Input: part model. Units: mm. Frame: model coordinates. Face numbers are marked on the shaded views. A direction names the side the tool comes from. Round coordinates to 2 decimals unless told otherwise and drop trailing zeros. Loops run counter-clockwise (first coordinate to the right, second up) from the corner with the lowest first, then second, coordinate; pieces in that order, holes last. Notation, with made-up numbers: (12, 27.5) -> (62, 27.5) arc R9 cw to (62, 40.5) -> close; hole circle Ø6 at (29, 66.5). An arc over 180 degrees is marked (long way). Answer as a JSON object with one key per item and string values. Group by question number.
Item 1: Draft query along Z for the marked faces 1, 2 and 3. Return one class per face: released by +Z, released by -Z, zero draft, split by the parting line, or undercut.
Item 2: Section query A-A on z = 0. Return loops of the section in (x, y).
Item 3: Pin query (flat end, axial travel): pin 1 (3 mm diameter, centred on y = 0, z = 0, fed in from -X); pin 2 (2 mm diameter, centred on x = 1, z = 6.5, fed in from -Y); pin 3 (1.5 mm diameter, centred on x = 1, z = -0.5, fed in from +Y); pin 4 (3 mm diameter, centred on x = 3.5, z = -7.5, fed in from +Y). Return the tip coordinate at first contact, or that it passes through.
Item 4: Material intervals for line 1 (Y direction, x = 1.6, z = 0); line 2 (Z direction, x = 2.75, y = -12); line 3 (Y direction, x = 3.3, z = 14), sorted ascending. Write a range as [from, to].
Item 5: Set-up query: the marked faces 4, 5 and 6. Return all of +Z, -Z, +X, -X, +Y, -Y with unobstructed straight access to the full face (end or side cutting, diameter ignored); none if empty.
from build123d import *

# Parameters (mm, degrees)
BASPROSKE_W        = 5
BASPROSKE_H        = 16
TOOTHCUT_DEPTH     = 24.173260453
TEETHCUTS_COUNT    = 30
TEETHCUTS_ANGLE    = 348
BORSKE_R           = 2.5
BORE_DEPTH         = 50.0000508
ESQUISSE1_R        = 3.356867485
BOSS_EXTRU_1_DEPTH = 5


with BuildPart() as part:
    # BasProSke → Base-Revolve (revolve)
    with BuildSketch(Plane(origin=(0, 0, 0), x_dir=(1, 0, 0), z_dir=(0, 1, 0)), mode=Mode.PRIVATE) as base_revolve_sk:
        with Locations((2.5, 8)):
            Rectangle(BASPROSKE_W, BASPROSKE_H)
    revolve(base_revolve_sk.sketch.rotate(Axis((-10, 0, 0), (1, 0, 0)), 180), axis=Axis((-10, 0, 0), (1, 0, 0)))

    # TooCutSke → ToothCut (cut, through all)
    with BuildSketch(Plane(origin=(0, 0, 0), x_dir=(0, 0, -1), z_dir=(1, 0, 0))):
        with BuildLine():
            ThreePointArc((0.466400716, 13.741086979), (0, 13.749), (-0.466400716, 13.741086979))
            ThreePointArc((-0.466400716, 13.741086979), (-0.819142092, 14.899954875), (-1.3974676, 15.964351834))
            ThreePointArc((-1.3974676, 15.964351834), (0, 16.0254), (1.3974676, 15.964351834))
            ThreePointArc((1.3974676, 15.964351834), (0.819142092, 14.899954875), (0.466400716, 13.741086979))
        make_face()
    toothcut = extrude(amount=TOOTHCUT_DEPTH, mode=Mode.SUBTRACT)

    # TeethCuts: ToothCut ×30 about axis
    teethcuts_axis = Axis((-10, 0, 0), (1, 0, 0))
    for i in range(1, TEETHCUTS_COUNT):
        add(toothcut.rotate(teethcuts_axis, i * TEETHCUTS_ANGLE / (TEETHCUTS_COUNT - 1)), mode=Mode.SUBTRACT)

    # BorSke → Bore (cut, symmetric)
    with BuildSketch(Plane(origin=(0, 0, 0), x_dir=(0, 0, -1), z_dir=(1, 0, 0))):
        with Locations(Location((0, 0, 0), (0, 0, 180))):
            Circle(BORSKE_R)
    extrude(amount=BORE_DEPTH, both=True, mode=Mode.SUBTRACT)

    # Esquisse1 → Boss.-Extru.1 (add)
    with BuildSketch(Plane(origin=(5, 0, 0), x_dir=(0, 0, -1), z_dir=(1, 0, 0))):
        Circle(ESQUISSE1_R)
        with BuildLine():
            Line((1.989182734, -1.514315704), (2.010613168, 1.485743817))
            ThreePointArc((2.010613168, 1.485743817), (-2.499936218, 0.017857885), (1.989182734, -1.514315704))
        make_face(mode=Mode.SUBTRACT)
    extrude(amount=-BOSS_EXTRU_1_DEPTH)


solid = part.part
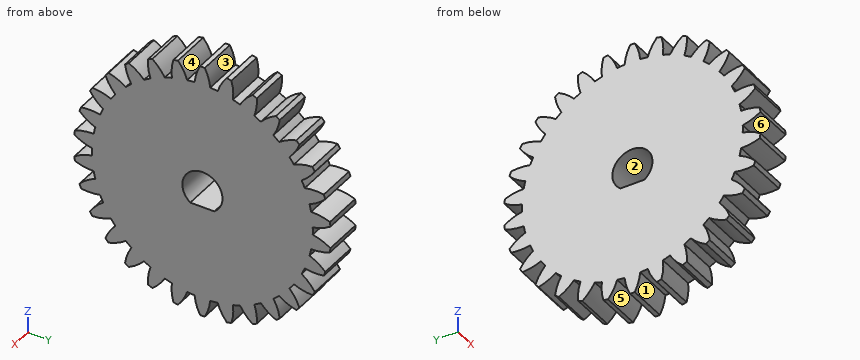
Solved:
{
 "1": {"face 1": "released by -Z", "face 2": "undercut", "face 3": "released by +Z"},
 "2": {"outline": "(0, -13.75) -> (5, -13.75) -> (5, -2.5) -> (0, -2.5) -> close; (0, 2.5) -> (5, 2.5) -> (5, 13.75) -> (0, 13.75) -> close"},
 "3": {"pin 1": "through", "pin 2": "y = -13.84", "pin 3": "y = 15.74", "pin 4": "y = 14"},
 "4": {"line 1": "[-13.75, -2.5], [2.5, 13.75]", "line 2": "[-10.58, -10.27], [-7.94, 7.94], [10.27, 10.58]", "line 3": "[-6.79, -5.46], [-3.85, -2.03], [-0.94, 0.94], [2.03, 3.85], [5.46, 6.79]"},
 "5": {"face 4": "+Z, +X, -X", "face 5": "-Z, +X, -X", "face 6": "+X, -X, -Y"}
}
